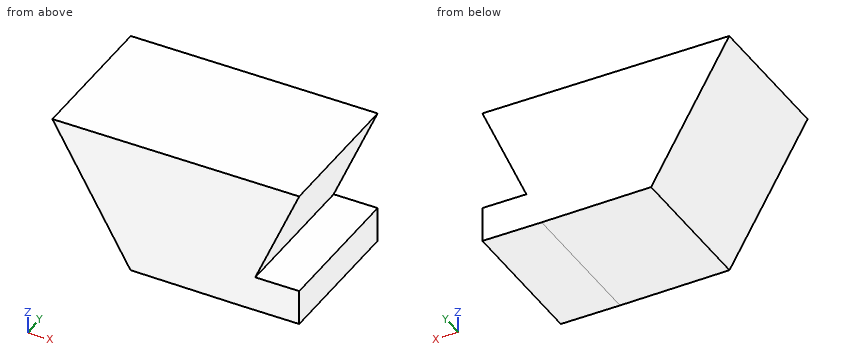
```python
from build123d import *

# Parameters (mm, degrees)
F1_DEPTH = 39.878


with BuildPart() as f1:
    # F0 (on Front) → F1 (new body)
    with BuildSketch(Plane.XZ):
        Polygon((14.062366, 8.441711), (-55.177242, 7.794467), (-33.257794, -30.311951), (-2.559891, -30.311951), (1.725662, -20.320477), align=None)
        Polygon((1.725662, -20.320477), (-2.559891, -30.311951), (14.062366, -30.156568), (14.062366, -20.205155), align=None)
    extrude(amount=F1_DEPTH)


solid = f1.part
```
Source: CAD feature listing. Evaluate the final solid. Frame: model axes, mm. Coordinates: 2 decimals unless noted, no trailing zeros. Loops run counter-clockwise (first coordinate to the right, second up) from the corner with the lowest first, then second, coordinate; pieces in that order, holes last. Notation, with made-up numbers: (14.25, 80) -> (43.25, 80) arc R35 cw to (43.25, 117) -> close; hole circle Ø1 at (39, -26.5). An arc over 180 degrees is marked (long way). One line per item, written item: value. Start each with the question number.
Q1. Section query C-C, the plane z = -2. Return the cut outline in (x, y).
Q2. Section query D-D, the plane x = -49.5. Return the cut outline in (y, z), and give its area (3 significant figures).
Q3. Section query A-A, the plane x = 9.5. Return the cut outline in (y, z).
Q4. Line query: line 1 along Z through (x, y) = (4, -29); line 2 along Z through (x, y) = (11.5, -15.5); line 3 along X through (y, z) = (-24.5, -8.5). Output: solid intervals per line, ascending.
Q5. Contact query for flat-ended pins moving along their axis: P1, Ø8, axis at y = -8, z = 0, coming from the +X side; P2, Ø8, axis at x = -35.5, y = -7, coming from the -Z side; P3, Ø4, axis at y = -28, z = -17, coming from the -X side; P4, Ø3, axis at y = -16, z = -23.5, coming from the -X side. Output: stop coordinate, or through.
Q6. Section query B-B, the plane y = -29. Return the cut outline in (x, z).
Results:
1. outline: (-49.54, -39.88) -> (9.58, -39.88) -> (9.58, 0) -> (-49.54, 0) -> close
2. outline: (-39.88, -2.08) -> (0, -2.08) -> (0, 7.85) -> (-39.88, 7.85) -> close
2. area: 396 mm^2
3. outline: (-39.88, -30.2) -> (0, -30.2) -> (0, -20.25) -> (-39.88, -20.25) -> close; (-39.88, -2.2) -> (0, -2.2) -> (0, 8.4) -> (-39.88, 8.4) -> close
4. line 1: -30.25 to -20.3, -15.02 to 8.35
4. line 2: -30.18 to -20.23, 2.47 to 8.42
4. line 3: -45.8 to 6.8
5. P1: x = 12.16
5. P2: z = -30.31
5. P3: x = -42.07
5. P4: x = -38.04
6. outline: (-55.18, 7.79) -> (-33.26, -30.31) -> (-2.56, -30.31) -> (14.06, -30.16) -> (14.06, -20.21) -> (1.73, -20.32) -> (14.06, 8.44) -> close
